Autodesk Inventor part; units mm, degrees
ref_plane "YZ Plane" through (0, 0, 0) normal (1, 0, 0) x (0, 1, 0)
ref_plane "XZ Plane" through (0, 0, 0) normal (0, 1, 0) x (-1, 0, 0)
ref_plane "XY Plane" through (0, 0, 0) normal (0, 0, 1) x (1, 0, 0)
sketch "Sketch1" plane through (0, 0, 0) normal (0, 1, 0) x (-1, 0, 0)
  line L0 (0, 0) -> (127, 0)
  line L1 (127, 0) -> (127, -101.6)
  line L2 (127, -101.6) -> (0, -101.6)
  line L3 (0, -101.6) -> (0, 0)
  dimension "d1" = 127
extrude "Extrusion1" add sketch "Sketch1" along normal blind 10
sketch "Sketch2" plane through (0, 10, 0) normal (0, 1, 0) x (1, 0, 0)
  line L0 (0, 0) -> (0, 101.6)
  line L1 (-5.9255, 8.3) -> (-61.9255, 8.3)
  line L2 (-61.9255, 8.3) -> (-61.9255, 93.3)
  line L3 (-61.9255, 93.3) -> (-5.9255, 93.3)
  line L4 (-5.9255, 93.3) -> (-5.9255, 8.3)
  line L5 (-5.9255, 8.3) -> (-61.9255, 93.3) construction
  line L6 (-61.9255, 8.3) -> (-5.9255, 93.3) construction
  line L7 (-126.4344, 50.8) -> (-96.4344, 50.8)
  circle A0 centre (-96.4344, 50.8) radius 3.5
  point P0 (-33.9255, 50.8)
  dimension "d5" = 56
  dimension "d6" = 85
  dimension "d7" = 30
  dimension "d8" = 7
extrude "Extrusion2" cut sketch "Sketch2" against normal through all contours A0
sketch "Sketch3" plane through (0, 10, 0) normal (0, 1, 0) x (1, 0, 0)
  line L0 (-5.9255, 8.3) -> (-61.9255, 93.3) construction
  line L1 (-61.9255, 8.3) -> (-5.9255, 93.3) construction
  line L2 (-126.4344, 50.8) -> (-96.4344, 50.8)
  circle A0 centre (-96.4344, 50.8) radius 3.5
  line L3 (-4.9255, 7.3) -> (-62.9255, 7.3)
  line L4 (-62.9255, 7.3) -> (-62.9255, 94.3)
  line L5 (-62.9255, 94.3) -> (-4.9255, 94.3)
  line L6 (-4.9255, 94.3) -> (-4.9255, 7.3)
  line L7 (-4.9255, 7.3) -> (-62.9255, 94.3) construction
  line L8 (-62.9255, 7.3) -> (-4.9255, 94.3) construction
  line L9 (-62.9255, 94.3) -> (-62.9255, 84.3)
  line L10 (-62.9255, 94.3) -> (-62.9255, 88.3)
  line L11 (-62.9255, 88.3) -> (-64.9255, 88.3)
  line L12 (-64.9255, 88.3) -> (-64.9255, 96.3)
  line L13 (-64.9255, 96.3) -> (-2.9255, 96.3)
  line L14 (-2.9255, 96.3) -> (-2.9255, 7.3)
  line L15 (-2.9255, 7.3) -> (-4.9255, 7.3)
  line L16 (-4.9255, 94.3) -> (-62.9255, 94.3)
  line L17 (-62.9255, 7.3) -> (-64.9255, 7.3)
  line L18 (-64.9255, 7.3) -> (-64.9255, 32.3)
  line L19 (-64.9255, 32.3) -> (-62.9255, 32.3)
  point P0 (-33.9255, 50.8)
  dimension "d13" = 30
  dimension "d14" = 7
  dimension "d20" = 6
  dimension "d21" = 2
  dimension "d22" = 8
  dimension "d23" = 62
  dimension "d24" = 2
  dimension "d25" = 25
extrude "Extrusion3" add sketch "Sketch3" along normal blind 10 contours L6 L5 L4 L11 L12 L13 L14 L15 | L17 L18 L19 L4
sketch "Sketch4" plane through (0, 10, 0) normal (0, 1, 0) x (1, 0, 0)
  circle A0 centre (-96.4344, 50.8) radius 3.5
  circle A1 centre (-96.4344, 50.8) radius 6.5
  point P0 (0, 0)
  dimension "d28" = 13
extrude "Extrusion4" cut sketch "Sketch4" against normal blind 4.5
sketch "Sketch5" plane through (0, 10, 0) normal (0, 1, 0) x (1, 0, 0)
  point P0 (0, 0)
properties part number "CraneBase"
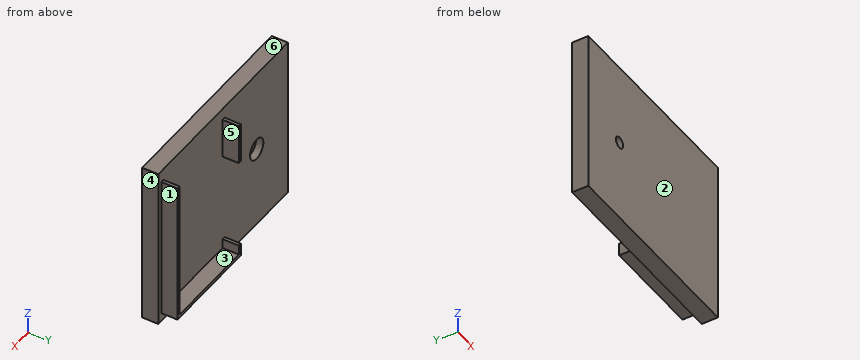
Geometry check sheet. Reference: the model listing, model coordinates, mm. Face numbers are marked on the shaded views. A direction names the side the tool comes from. Round coordinates to 2 decimals unless told otherwise and drop trailing zeros. Order: outer loops, then holes, each group sorted by start corner. A loop starts at its lowest first (then second) coordinate and runs counter-clockwise, first axis right, second up. Notation, with made-up numbers: (18.5, 73.5) -> (38.5, 73.5) arc R15 cw to (38.5, 97.5) -> close; hole circle Ø5 at (0, -23). An arc over 180 degrees is marked (long way). Return JSON: item names as keys, results as strings. Group by question number.
Q1. Release check for a two-part mould opening along X. For the marked faces 4, 5 and 6 record: released by +X, released by -X, zero draft, split by the parting line, or undercut.
Q2. Material ranges on probe 1 along X at (y, z) = (8.1, -50.8); probe 2 along Z at (x, y) = (-64, 13.75); probe 3 along X at (y, z) = (2.75, -50.8), recorded low to high. Write a range as from..to.
Q3. Section check A-A, the plane y = 17. Record the boundary of the cut face in (x, z).
Q4. Tool access check on the marked faces 1, 2 and 3. Record the directions out of +Z, -Z, +X, -X, +Y, -Y that give a thin tool (end or side, any length) a straight path to the whole face; none if there is none.
Q5. Gauge pin test, flat ends, axial feed: pin 1 (11 mm diameter, centred on x = -46, y = 16.5, fed in from -Z); pin 2 (11 mm diameter, centred on y = 17, z = -20, fed in from +X); pin 3 (0.6 mm diameter, centred on x = -63.5, y = 13.5, fed in from +Z). Record the tip position at first contact, or that the pin passes through.
Q6. Section check D-D, the plane x = -20. Record the boundary of the cut face in (y, z), plus the area to 3 significant figures.
Q7. Section check C-C, the plane z = -85. Record the boundary of the cut face in (x, y).
Q8. Section check B-B, the plane z = -50.8. Record the boundary of the cut face in (x, y).
Numbers:
{
 "1": {"face 4": "released by +X", "face 5": "undercut", "face 6": "zero draft"},
 "2": {"probe 1": "-127..-102.93, -89.93..0", "probe 2": "-96.3..-88.3, -32.3..-7.3", "probe 3": "-127..-99.93, -92.93..0"},
 "3": {"outline": "(-64.93, -96.3) -> (-2.93, -96.3) -> (-2.93, -7.3) -> (-4.93, -7.3) -> (-4.93, -94.3) -> (-62.93, -94.3) -> (-62.93, -88.3) -> (-64.93, -88.3) -> close; (-64.93, -32.3) -> (-62.93, -32.3) -> (-62.93, -7.3) -> (-64.93, -7.3) -> close"},
 "4": {"face 1": "+Z, -Z, +X, +Y", "face 2": "+Z, -Z, +X, -X, -Y", "face 3": "+Z, +Y"},
 "5": {"pin 1": "z = -96.3", "pin 2": "x = -2.93", "pin 3": "z = -7.3"},
 "6": {"outline": "(0, -101.6) -> (10, -101.6) -> (10, -96.3) -> (20, -96.3) -> (20, -94.3) -> (10, -94.3) -> (10, 0) -> (0, 0) -> close", "area": "1,040 mm^2"},
 "7": {"outline": "(-127, 0) -> (0, 0) -> (0, 10) -> (-2.93, 10) -> (-2.93, 20) -> (-4.93, 20) -> (-4.93, 10) -> (-127, 10) -> close"},
 "8": {"outline": "(-127, 0) -> (-99.93, 0) -> (-99.93, 5.5) -> (-102.93, 5.5) -> (-102.93, 10) -> (-127, 10) -> close; (-92.93, 0) -> (0, 0) -> (0, 10) -> (-2.93, 10) -> (-2.93, 20) -> (-4.93, 20) -> (-4.93, 10) -> (-89.93, 10) -> (-89.93, 5.5) -> (-92.93, 5.5) -> close"}
}
